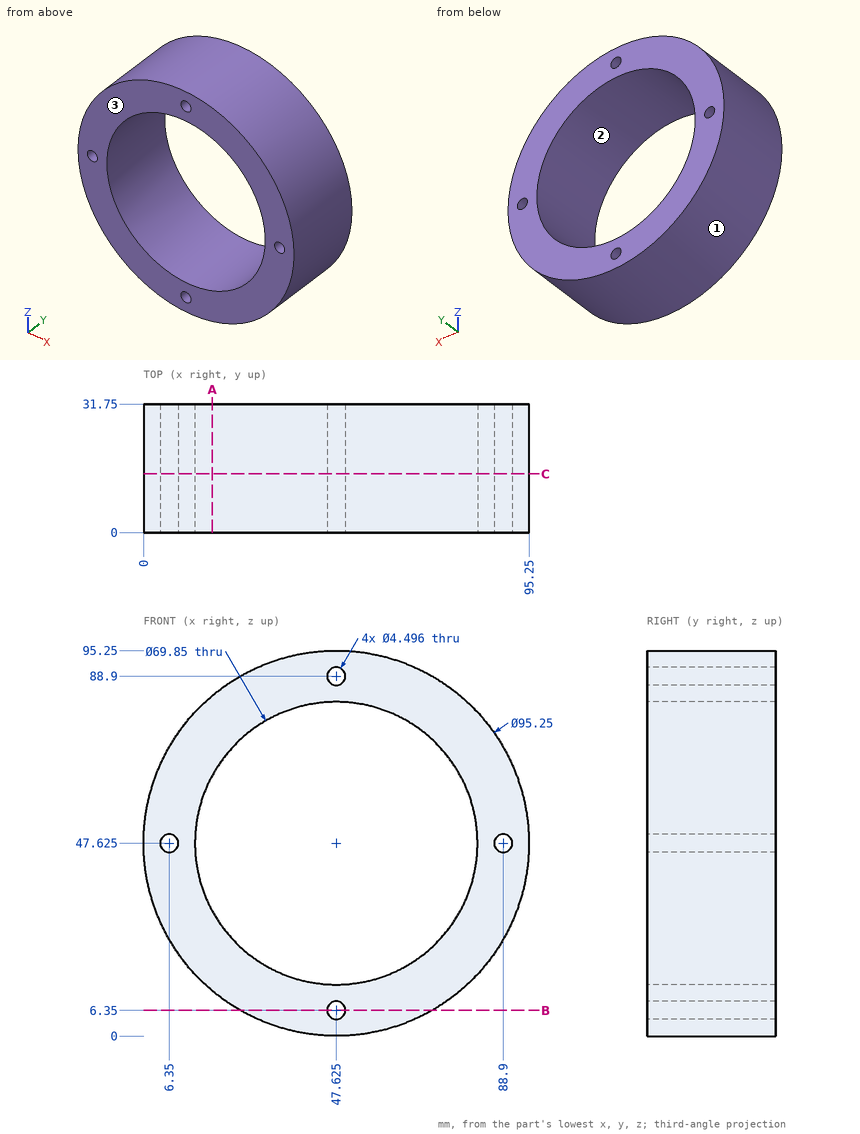
Geometry check sheet. Reference: drawing and pictorial views, mm from the part's lowest x, y, z. Give positions to 0.01 mm unless a question says otherwise; leave off trailing zeros. Order: outer loops, then holes, each group sorted by start corner. A loop starts at its lowest first (then second) coordinate and runs counter-clockwise, first axis right, second up. Notation, with made-up numbers: (70.5, 47.25) - (120.5, 47.25) arc R31 cw to (120.5, 74.25) - close; hole circle Ø6 at (1, 30.5). An arc over 180 degrees is marked (long way). Use one line per item in the form item = value.
1) Sectioned sample at B-B (z = 6.35). Record the boundary of the cut face in (x, y).
Working result:
outline = (23.87, 0) - (45.38, 0) - (45.38, 31.75) - (23.87, 31.75) - close; (49.87, 0) - (71.38, 0) - (71.38, 31.75) - (49.87, 31.75) - close
2) Depth check by flat-ended pin: pin 1 Ø12 at (x, y) = (71.5, 25) entering from -Z; pin 2 Ø2 at (x, y) = (74, 13.5) entering from +Z; pin 3 Ø12 at (x, y) = (39, 11) entering from -Z. Enter the tip coordinate at first touch or a pass-through.
Working result:
pin_1 = 3.48
pin_2 = 87.93
pin_3 = 0.07
3) Draft check along X on the marked faces 1, 2 and 3. Enter one of: released by +X, released by -X, zero draft, split by the parting line, or undercut.
Working result:
face_1 = split by the parting line
face_2 = undercut
face_3 = zero draft
4) Sectioned sample at C-C (y = 14.5). Count the separate pieces of the cut face and the enclosed holes in it, and give its area (3 significant figures).
Working result:
separate_pieces = 1
enclosed_holes = 5
area = 3,230 mm^2
5) Material ranges on probe 1 along X at (y, z) = (9, 30.5) (1 decimal); probe 2 along X at (y, z) = (3, 31.5) (1 decimal); probe 3 along Z at (x, y) = (34, 3.5), recorded low to high. Write a range as from..to.
Working result:
probe_1 = 3.2..17.2, 78.1..92.1
probe_2 = 2.8..16.6, 78.6..92.4
probe_3 = 1.99..15.47, 79.78..93.26
6) Sectioned sample at A-A (x = 17). Record the boundary of the cut face in (y, z), and give its area (3 significant figures).
Working result:
outline = (0, 11.15) - (31.75, 11.15) - (31.75, 30.84) - (0, 30.84) - close; (0, 64.41) - (31.75, 64.41) - (31.75, 84.1) - (0, 84.1) - close
area = 1,250 mm^2
